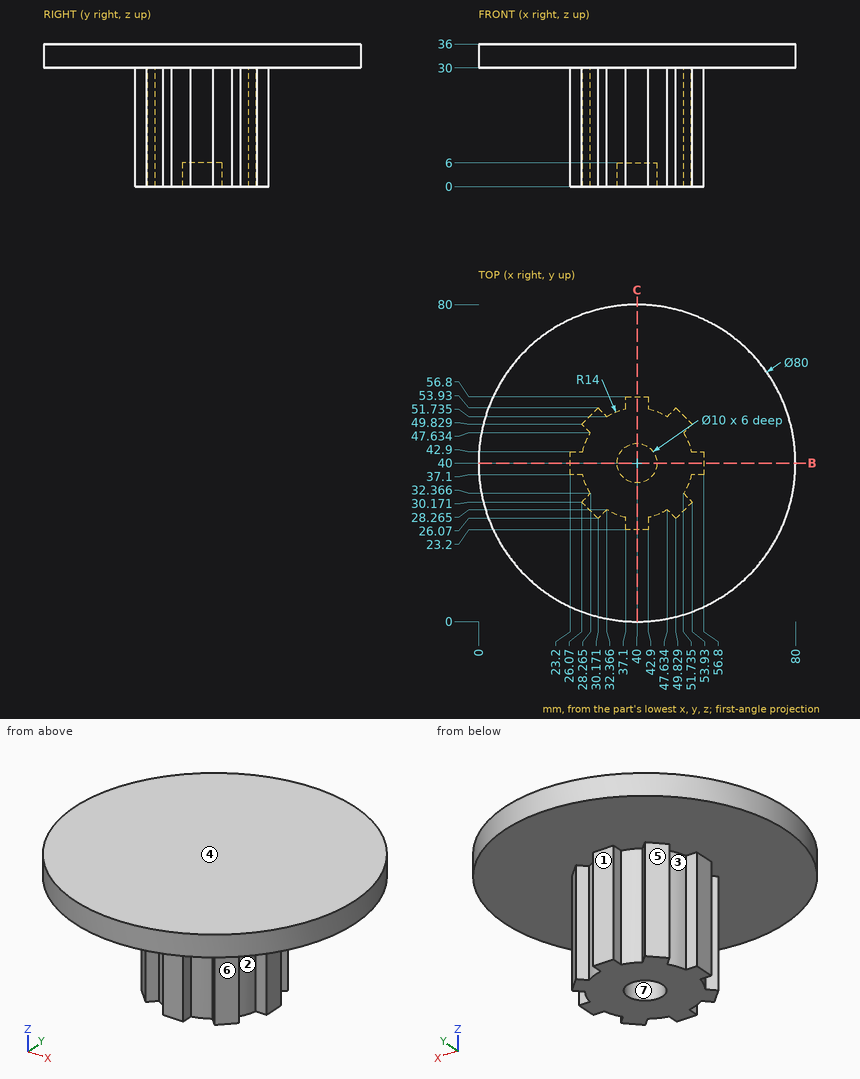
The figure shows three views and two pictorial views of one solid part (mm, origin at its lowest corner). Answer the questions. A direction names the side the tool comes from. Round coordinates to 2 decimals unless told otherwise and drop trailing zeros. Loops run counter-clockwise (first coordinate to the right, second up) from the corner with the lowest first, then second, coordinate; pieces in that order, holes last. Notation, with made-up numbers: (33, 85) -> (84, 85) arc R21 cw to (84, 103) -> close; hole circle Ø1 at (18, 70.5). An arc over 180 degrees is marked (long way). Use one line per item in the form item = value.
(1) A tool of negligible diameter and unlimited length cuts with its end or side. For the marked faces 1, 2 and 3, from which of +Z, -Z, +X, -X, +Y, -Y can it reach the whole face along a straight path? Write none if from no direction.
Answer list:
face_1 = -Z, +X, -X, +Y
face_2 = -Z, +X
face_3 = -Z, -X
(2) Flat-ended cylindrical pins translate along their axes: P1, Ø6.5, axis at y = 40.5, z = 10, coming from the -X side; P2, Ø4.5, axis at y = 39.5, z = 20.5, coming from the +X side; P3, Ø6.5, axis at x = 41, z = 8, coming from the +Y side. Find the tip coordinate at first contact, or state that the pin passes through.
Answer list:
P1 = 23.2
P2 = 56.8
P3 = 56.8
(3) Straight lines are drawn through the part: line 1 (Z direction, x = 28, y = 13.5); line 2 (X direction, y = 39.5, z = 32); line 3 (Y direction, x = 25.5, z = 10). For each, find the intervals that lie inside material, in ascending order.
Answer list:
line_1 = 30 to 36
line_2 = 0 to 80
line_3 = 37.1 to 42.9
(4) Find section B-B on y = 40. Give the vertices of the cut face in (x, z), then the cut area to 3 significant figures.
Answer list:
outline = (0, 30) -> (23.2, 30) -> (23.2, 0) -> (35, 0) -> (35, 6) -> (45, 6) -> (45, 0) -> (56.8, 0) -> (56.8, 30) -> (80, 30) -> (80, 36) -> (0, 36) -> close
area = 1,430 mm2
(5) For a pull along X with two mould halves and no side action, classify the marked faces 4, 5, 6 and 7 as released by +X, released by -X, zero draft, split by the parting line, or undercut.
Answer list:
face_4 = zero draft
face_5 = released by -X
face_6 = released by +X
face_7 = undercut
